```python
from build123d import *

# Parameters (mm, degrees)
F0_W      = 152.4
F0_H      = 190.5
F1_DEPTH  = 127
F2_T      = -2.54
F3_W      = 63.5
F3_H      = 63.5
F4_DEPTH  = 38.1
F5_R      = 5.08
F7_DEPTH  = 177.8
F8_R      = 38.1
F9_DEPTH  = 12.7
F11_DEPTH = 25.4
F12_R     = 38.1
F12_R_2   = 12.7
F13_DEPTH = 12.7


with BuildPart() as f1:
    # F0 (on Top) → F1 (new body)
    with BuildSketch(Plane.XY):
        with Locations((-1.2951251119, 11.9785609818)):
            Rectangle(F0_W, F0_H)
    extrude(amount=F1_DEPTH)

    # F2
    f2_openings = [f1.faces().sort_by_distance(p)[0] for p in [
        (-1.295125, 11.978561, 127),
    ]]
    offset(amount=F2_T, openings=f2_openings)

    # F3 (on face) → F4 (join)
    with BuildSketch(Plane.XZ.offset(83.2714390182)):
        with Locations((3.0893431157, 31.75)):
            Rectangle(F3_W, F3_H)
    extrude(amount=F4_DEPTH)

    # F5
    f5_edges = [f1.edges().sort_by_distance(p)[0] for p in [
        (-28.660657, -121.371439, 31.75),
        (34.839343, -121.371439, 31.75),
        (3.089343, -121.371439, 63.5),
        (34.839343, -102.321439, 63.5),
        (-28.660657, -102.321439, 63.5),
        (3.089343, -121.371439, 0),
        (-28.660657, -102.321439, 0),
        (34.839343, -102.321439, 0),
    ]]
    fillet(f5_edges, radius=F5_R)

    # F6 (on face) → F7 (join)
    with BuildSketch(Plane(origin=(-77.4951251119, 0, 0), x_dir=(0, -1, 0), z_dir=(-1, 0, 0))):
        with BuildLine():
            ThreePointArc((20.8495695472, 0), (33.5495695472, -12.7), (46.2495695472, 0))
            Line((46.2495695472, 0), (20.8495695472, 0))
        make_face()
        with BuildLine():
            Line((-86.981655252, 0), (-61.581655252, 0))
            ThreePointArc((-61.581655252, 0), (-74.281655252, 12.7), (-86.981655252, 0))
        make_face()
        with BuildLine():
            Line((20.8495695472, 0), (46.2495695472, 0))
            ThreePointArc((46.2495695472, 0), (33.5495695472, 12.7), (20.8495695472, 0))
        make_face()
        with BuildLine():
            ThreePointArc((-86.981655252, 0), (-74.281655252, -12.7), (-61.581655252, 0))
            Line((-61.581655252, 0), (-86.981655252, 0))
        make_face()
    extrude(amount=-F7_DEPTH)

    # F8 (on face) → F9 (join)
    with BuildSketch(Plane.YZ.offset(100.3048748881)):
        with Locations((-33.5495695472, 0)):
            Circle(F8_R)
        with Locations((74.2916837335, 0)):
            Circle(F8_R)
    extrude(amount=F9_DEPTH)

    # F10 (on face) → F11 (join)
    with BuildSketch(Plane(origin=(-77.4951251119, 0, 0), x_dir=(0, -1, 0), z_dir=(-1, 0, 0))):
        with BuildLine():
            ThreePointArc((46.2495695472, 0), (33.5495695472, 12.7), (20.8495695472, 0))
            ThreePointArc((20.8495695472, 0), (33.5495695472, -12.7), (46.2495695472, 0))
        make_face()
        with BuildLine():
            ThreePointArc((-86.981655252, 0), (-74.281655252, -12.7), (-61.581655252, 0))
            ThreePointArc((-61.581655252, 0), (-74.281655252, 12.7), (-86.981655252, 0))
        make_face()
    extrude(amount=F11_DEPTH)

    # F12 (on face) → F13 (join)
    with BuildSketch(Plane(origin=(-102.8951251119, 0, 0), x_dir=(0, -1, 0), z_dir=(-1, 0, 0))):
        with Locations((-74.281655252, 0)):
            Circle(F12_R)
        with Locations((-74.281655252, 0)):
            Circle(F12_R_2, mode=Mode.SUBTRACT)
        with Locations((33.9739844203, 0)):
            Circle(F12_R)
        with Locations((-74.281655252, 0)):
            Circle(F12_R_2)
    extrude(amount=F13_DEPTH)


solid = f1.part
```
Verification items for the finished model (mm, model axes). A direction names the side the tool comes from. Coordinates: 2 decimals unless noted, no trailing zeros. Loops run counter-clockwise (first coordinate to the right, second up) from the corner with the lowest first, then second, coordinate; pieces in that order, holes last. Notation, with made-up numbers: (19.5, 28.25) -> (34.5, 28.25) arc R32 cw to (34.5, 64.25) -> close; hole circle Ø7 at (45.5, 86). An arc over 180 degrees is marked (long way). Answer in a Markdown table with one row per item. Add a question column.
1. Material ranges on probe 1 along X at (y, z) = (54, -17); probe 2 along Y at (x, z) = (-0.5, 68); probe 3 along X at (y, z) = (101.5, 107), recorded low to high. Write a range as [from, to].
2. Section check D-D, the plane z = 96. Enter the section's corners in (x, y), then the cut area to 3 significant figures.
3. Section check B-B, the plane x = -3.5. Enter the section's corners in (y, z).
4. Section check C-C, the plane y = -12. Enter the section's corners in (x, z).
5. Draft check along Y on faces 4 (the face through (-2, 97, 0)), 5 (the face through (-109.16, 37.94, 11.44)), 6 (the face through (-2, -83.271, 77)). Enter one of: +Y half, -Y half, draft (parallel to the pull), parting line (faces both ways), or undercut.
6. Section check A-A, the plane z = 30.5. Give the number of separate pieces and of enclosed holes in the cut face, then the cut area to 3 significant figures.
7. Depth check by flat-ended pin: P1, Ø12, axis at y = 40.5, z = 40.5, coming from the +X side; P2, Ø3, axis at y = -87, z = 47.5, coming from the +X side; P3, Ø3, axis at x = 46.5, y = -61.5, coming from the -Z side; P4, Ø20, axis at x = 29.5, y = 100, coming from the +Z side. Enter the tip coordinate at first touch or a pass-through.
8. Access from +Z, -Z, +X, -X, +Y, -Y to the whole of each face (thin tool, end or side, straight path). Record for faces 1 (the face through (100.305, -43, 9)), 2 (the face through (106.566, 2.791, 11.444)), 3 (the face through (-2, 21, 2.54)).
Derived:
| question | item | result |
|---|---|---|
| 1 | probe 1 | x = [-115.6, -102.9], [100.3, 113] |
| 1 | probe 2 | y = [-83.27, -80.73], [104.69, 107.23] |
| 1 | probe 3 | x = [-77.5, -74.96], [72.36, 74.9] |
| 2 | outline | (-77.5, -83.27) -> (74.9, -83.27) -> (74.9, 107.23) -> (-77.5, 107.23) -> close; hole (-74.96, -80.73) -> (72.36, -80.73) -> (72.36, 104.69) -> (-74.96, 104.69) -> close |
| 2 | area | 1,720 mm² |
| 3 | outline | (-121.37, 5.08) arc R5.08 ccw to (-116.29, 0) -> (-46.25, 0) arc R12.7 ccw to (-20.85, 0) -> (61.58, 0) arc R12.7 ccw to (86.98, 0) -> (107.23, 0) -> (107.23, 127) -> (104.69, 127) -> (104.69, 2.54) -> (86.73, 2.54) arc R12.7 ccw to (61.84, 2.54) -> (-21.11, 2.54) arc R12.7 ccw to (-45.99, 2.54) -> (-80.73, 2.54) -> (-80.73, 127) -> (-83.27, 127) -> (-83.27, 63.5) -> (-116.29, 63.5) arc R5.08 ccw to (-121.37, 58.42) -> close |
| 4 | outline | (-115.6, -31.12) -> (-102.9, -31.12) -> (-102.9, 31.12) -> (-115.6, 31.12) -> close; (-77.5, 0) -> (74.9, 0) -> (74.9, 127) -> (72.36, 127) -> (72.36, 2.54) -> (-74.96, 2.54) -> (-74.96, 127) -> (-77.5, 127) -> close; (100.3, -31.42) -> (113, -31.42) -> (113, 31.42) -> (100.3, 31.42) -> close |
| 5 | face 4 | draft |
| 5 | face 5 | undercut |
| 5 | face 6 | -Y half |
| 6 | separate pieces | 5 |
| 6 | enclosed holes | 1 |
| 6 | area | 6,440 mm² |
| 7 | P1 | stops at x = 74.9 |
| 7 | P2 | stops at x = 34.84 |
| 7 | P3 | stops at z = 0 |
| 7 | P4 | stops at z = 127 |
| 8 | face 1 | none |
| 8 | face 2 | +X |
| 8 | face 3 | +Z |
